Read the model definition and answer for the solid it produces. Units are mm, in the model's axes. A direction names the side the tool comes from. Give positions to 0.01 mm unless a question says otherwise; leave off trailing zeros. Write each loop counter-clockwise with the first axis right and the second up, starting at its lowest first coordinate (ties: lowest second). Pieces come first, ordered by that corner, then holes. Notation, with made-up numbers: M 68.25,27 L 116.25,27 A35 cw 116.25,59 Z; hole C 70.5,-38.75 d4. An arc over 180 degrees is marked long. Answer as CSV lines item,"result". Start each with the question number.
```python
from build123d import *

# Parameters (mm, degrees)
SKETCH1_W               = 730
SKETCH1_H               = 150
BASE_FLANGE1_DEPTH      = 2.5
EDGE_FLANGE1_DEPTH      = 730
EDGE_FLANGE1_BEND_DEPTH = 730
CUT_EXTRUDE1_DEPTH      = 418.461567093
CUT_EXTRUDE1_DEPTH_BACK = 418.461567093
SKETCH12_R              = 434
SKETCH13_R              = 22.5
CUT_EXTRUDE2_DEPTH      = 10
CUT_EXTRUDE3_DEPTH      = 396.173746598
CUT_EXTRUDE3_DEPTH_BACK = 396.173746598
SKETCH14_W              = 631.337566112
SKETCH14_H              = 273.157514278
CUT_EXTRUDE4_DEPTH      = 396.173746598
CUT_EXTRUDE4_DEPTH_BACK = 396.173746598
CUT_EXTRUDE5_DEPTH      = 400.448552929


# Sheet-metal steps are written as plain solids
with BuildPart() as part:
    # Sketch1 → Base-Flange1 (new body)
    with BuildSketch(Plane(origin=(0, 0, 0), x_dir=(0, 0, -1), z_dir=(1, 0, 0))):
        Rectangle(SKETCH1_W, SKETCH1_H)
    extrude(amount=-BASE_FLANGE1_DEPTH)

    # Edge-Flange1 section (across the edge) → Edge-Flange1 (add)
    with BuildSketch(Plane(origin=(-2.5, 75.2, 365), x_dir=(0, -1, 0), z_dir=(0, 0, -1))):
        with BuildLine():
            Line((-2.5, 0.2), (-2.5, 127.5))
            Line((-2.5, 127.5), (0, 127.5))
            Line((0, 127.5), (0, 0.2))
            ThreePointArc((0, 0.2), (0.058578644, 0.058578644), (0.2, 0))
            Line((0.2, 0), (0.2, -2.5))
            ThreePointArc((0.2, -2.5), (-1.709188309, -1.709188309), (-2.5, 0.2))
        make_face()
    extrude(amount=EDGE_FLANGE1_DEPTH)

    # Edge-Flange1 section 2 (across the edge) → Edge-Flange1 bend (add)
    with BuildSketch(Plane(origin=(-2.5, -75.2, -365), x_dir=(0, 1, 0), z_dir=(0, 0, 1))):
        with BuildLine():
            Line((-2.5, 0.2), (-2.5, 127.5))
            Line((-2.5, 127.5), (0, 127.5))
            Line((0, 127.5), (0, 0.2))
            ThreePointArc((0, 0.2), (0.058578644, 0.058578644), (0.2, 0))
            Line((0.2, 0), (0.2, -2.5))
            ThreePointArc((0.2, -2.5), (-1.709188309, -1.709188309), (-2.5, 0.2))
        make_face()
    extrude(amount=EDGE_FLANGE1_BEND_DEPTH)

    # Sketch12 → Cut-Extrude1 (cut, two sides: drawn at the far end of the back side and taken through both)
    with BuildSketch(Plane(origin=(0, 77.7, 0), x_dir=(1, 0, 0), z_dir=(0, 1, 0)).offset(-CUT_EXTRUDE1_DEPTH_BACK)):
        with Locations((-470, 85)):
            Circle(SKETCH12_R)
    extrude(amount=CUT_EXTRUDE1_DEPTH + CUT_EXTRUDE1_DEPTH_BACK, mode=Mode.SUBTRACT)

    # Sketch13 → Cut-Extrude2 (cut)
    with BuildSketch(Plane(origin=(0, 0, 0), x_dir=(0, 0, -1), z_dir=(1, 0, 0))):
        with Locations((265, 0)):
            Circle(SKETCH13_R)
        with Locations((-290, 0)):
            Circle(SKETCH13_R)
    extrude(amount=-CUT_EXTRUDE2_DEPTH, mode=Mode.SUBTRACT)

    # Sketch14 → Cut-Extrude3 (cut, two sides: drawn at the far end of the back side and taken through both)
    with BuildSketch(Plane(origin=(0, 0, 0), x_dir=(0, 0, -1), z_dir=(1, 0, 0)).offset(-CUT_EXTRUDE3_DEPTH_BACK)):
        with Locations((-126.629311255, -14.019673746)):
            Rectangle(SKETCH14_W, SKETCH14_H)
    extrude(amount=CUT_EXTRUDE3_DEPTH + CUT_EXTRUDE3_DEPTH_BACK, mode=Mode.SUBTRACT)

    # Sketch15 → Cut-Extrude4 (cut, two sides: drawn at the far end of the back side and taken through both)
    with BuildSketch(Plane(origin=(0, 0, 0), x_dir=(0, 0, -1), z_dir=(1, 0, 0)).offset(-CUT_EXTRUDE4_DEPTH_BACK)):
        with BuildLine():
            Line((302.266550641, 80.822052704), (310.532003477, 105.351783703))
            Line((310.532003477, 105.351783703), (400.668447303, 94.566226322))
            Line((400.668447303, 94.566226322), (380.252927975, -108.048173048))
            Line((380.252927975, -108.048173048), (291.286888445, -85.029403714))
            ThreePointArc((291.286888445, -85.029403714), (353.805609642, -5.879089735), (302.266550641, 80.822052704))
        make_face()
    extrude(amount=CUT_EXTRUDE4_DEPTH + CUT_EXTRUDE4_DEPTH_BACK, mode=Mode.SUBTRACT)

    # Sketch16 → Cut-Extrude5 (cut, through all)
    with BuildSketch(Plane.XZ.offset(77.7)):
        with BuildLine():
            Line((-39.289490613, -183.753349909), (-75.528167694, -178.562999568))
            Line((-75.528167694, -178.562999568), (-125.004878412, -316.53047916))
            Line((-125.004878412, -316.53047916), (-101.585534734, -324.928922734))
            ThreePointArc((-101.585534734, -324.928922734), (-63.999675541, -257.181937871), (-39.289490613, -183.753349909))
        make_face()
    extrude(amount=-CUT_EXTRUDE5_DEPTH, mode=Mode.SUBTRACT)


solid = part.part
```
1. Find the intervals of material crossed by line 1 (Y direction, x = -27, z = -272.5); line 2 (Y direction, x = -1.8, z = -265); line 3 (X direction, y = -46.5, z = -203), in increasing order. Write a range as [from, to].
2. Find section C-C on z = -265. Determine the outline of the cut face in (x, y).
3. Find section A-A on x = -24.5. Determine the outline of the cut face in (y, z).
4. Find section D-D on z = -219. Determine the outline of the cut face in (x, y).
5. Find section B-B on y = 0. Determine the outline of the cut face in (x, z), then the cut area to 3 significant figures.
6. For faces 1 (the face through (-62.52, 76.43, -253.79)), 2 (the face through (-39, 75.2, -264)), determine the directions among +Z, -Z, +X, -X, +Y, -Y from which every point of the face is accessible in a straight line to the end or side of a thin tool.
7. Given pin 1 (6 mm diameter, centred on y = -41, z = -265.5, fed in from -X), flat-ended and moving along its own axis, determine where the tip first touches the part or whether it passes through.
Computed:
1,line 1,"y = [-77.7, -75.2], [75.2, 77.7]"
1,line 2,"y = [-77.55, -22.5], [22.5, 77.55]"
1,line 3,"x = [-2.5, 0]"
2,outline,"M -67.54,-77.7 L -2.7,-77.7 A2.7 ccw 0,-75 L 0,-22.5 L -2.5,-22.5 L -2.5,-75 A0.2 cw -2.7,-75.2 L -67.54,-75.2 Z; M -67.54,75.2 L -2.7,75.2 A0.2 cw -2.5,75 L -2.5,22.5 L 0,22.5 L 0,75 A2.7 ccw -2.7,77.7 L -67.54,77.7 Z"
3,outline,"M -77.7,-308.4 A89 ccw -75.2,-312.6 L -75.2,-189.04 L -77.7,-189.04 Z; M 75.2,-312.6 A89 ccw 77.7,-308.4 L 77.7,-189.04 L 75.2,-189.04 Z"
4,outline,"M -49.3,-77.7 L -2.7,-77.7 A2.7 ccw 0,-75 L 0,75 A2.7 ccw -2.7,77.7 L -49.3,77.7 L -49.3,75.2 L -2.7,75.2 A0.2 cw -2.5,75 L -2.5,-75 A0.2 cw -2.7,-75.2 L -49.3,-75.2 Z"
5,outline,"M -2.5,-354 L 0,-354 L 0,-287.5 L -2.5,-287.5 Z; M -2.5,-242.5 L 0,-242.5 L 0,-189.04 L -2.5,-189.04 Z"
5,area,"300 mm^2"
6,face 1,"+Z, -X, +Y, -Y"
6,face 2,"+Z, -Z, -X"
7,pin 1,"stops at x = -2.5"
